Study the drawing (mm; zero at the part's minimum x, y, z) and answer. A direction names the side the tool comes from. Give positions to 0.01 mm unless a question says otherwise; leave off trailing zeros. Write each loop counter-clockwise with the first axis right and the second up, starting at its lowest first coordinate (ties: lowest second). Pieces come first, ordered by that corner, then holes.
1) Find section A-A (y = 10). Determine the outline of the cut face in (x, z).
2) Given pin 1 Ø1.6 at (x, z) = (31, 11.5) entering from -Y; pin 2 Ø12 at (x, z) = (10, 3.5) entering from -Y; pin 3 Ø2 at (x, y) = (31, 1.5) entering from -Z; pin 4 Ø10 at (x, y) = (10.5, 9) entering from +Z, each flat-ended and moving along its own axis, determine where each tip first touches the part or whether it passes through.
3) Straight lines are drawn through the part: probe 1 along Y at (x, z) = (10, 0.4); probe 2 along X at (y, z) = (5, 19.5); probe 3 along Z at (x, y) = (17, 9.75). For each, find the intervals that lie inside material, in ascending order.
4) A tool of negligible diameter and unlimited length cuts with its end or side. For the marked faces 1 and 2, from which of +Z, -Z, +X, -X, +Y, -Y can it reach the whole face along a straight path? Write none if from no direction.
5) Find section B-B (z = 22). Determine the outline of the cut face in (x, y), plus the area to 3 significant figures.
6) Find section C-C (x = 10). Determine the outline of the cut face in (y, z), plus the area to 3 significant figures.
7) Find section D-D (y = 17.25). Determine the outline of the cut face in (x, z).
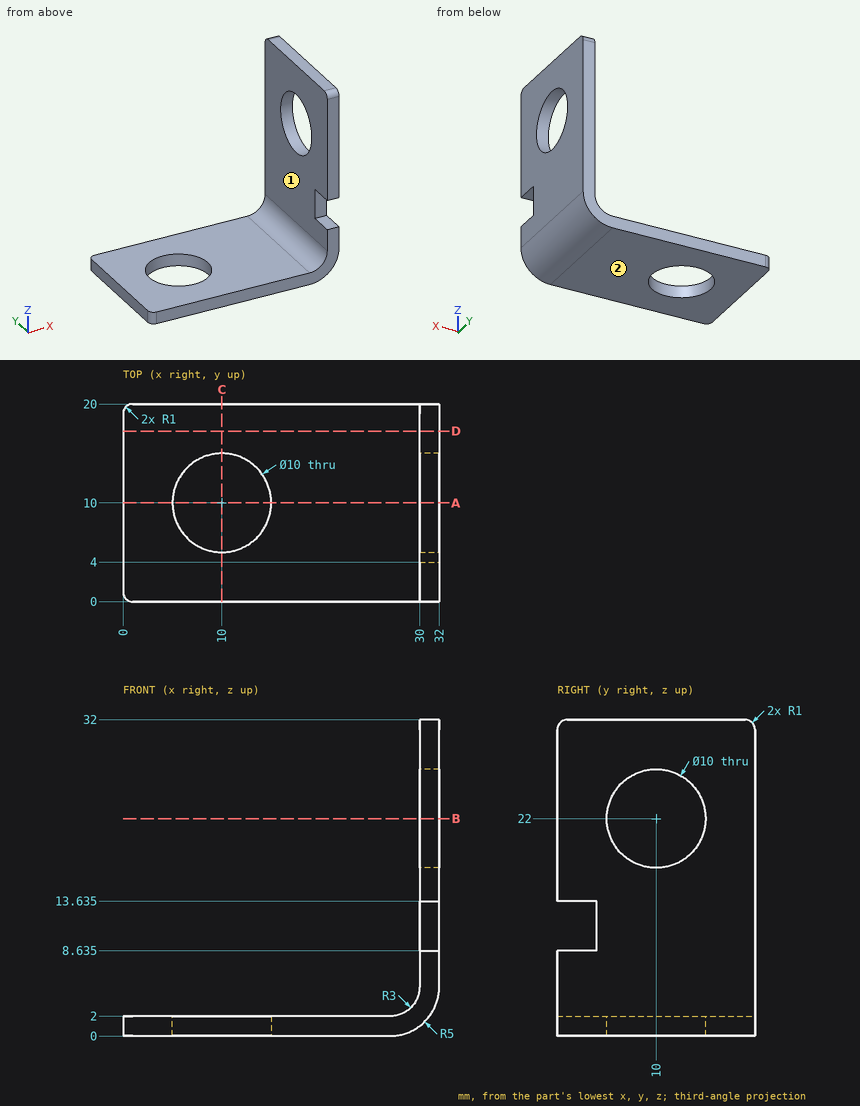
Results:
1. outline: (0, 0) - (5, 0) - (5, 2) - (0, 2) - close; (15, 0) - (27, 0) arc R5 ccw to (32, 5) - (32, 17) - (30, 17) - (30, 5) arc R3 cw to (27, 2) - (15, 2) - close; (30, 27) - (32, 27) - (32, 32) - (30, 32) - close
2. pin 1: stops at y = 4
2. pin 2: stops at y = 0
2. pin 3: stops at z = 1
2. pin 4: stops at z = 2
3. probe 1: y = 0 to 5, 15 to 20
3. probe 2: x = 30 to 32
3. probe 3: z = 0 to 2
4. face 1: +Z, -X, +Y, -Y
4. face 2: -Z, +X, -X, +Y, -Y
5. outline: (30, 0) - (32, 0) - (32, 5) - (30, 5) - close; (30, 15) - (32, 15) - (32, 20) - (30, 20) - close
5. area: 20.0 mm2
6. outline: (0, 0) - (5, 0) - (5, 2) - (0, 2) - close; (15, 0) - (20, 0) - (20, 2) - (15, 2) - close
6. area: 20.0 mm2
7. outline: (0, 0) - (27, 0) arc R5 ccw to (32, 5) - (32, 32) - (30, 32) - (30, 5) arc R3 cw to (27, 2) - (0, 2) - close
